```python
from build123d import *

# Parameters (mm, degrees)
CROQUIS1_R              = 3.25
SALIENTE_EXTRUIR1_DEPTH = 1.2
CROQUIS2_R              = 1.75
SALIENTE_EXTRUIR2_DEPTH = 22.1
REDONDEO2_R             = 0.4


with BuildPart() as part:
    # Croquis1 → Saliente-Extruir1 (new body)
    with BuildSketch(Plane.XY):
        Circle(CROQUIS1_R)
    extrude(amount=SALIENTE_EXTRUIR1_DEPTH)

    # Croquis2 → Saliente-Extruir2 (add)
    with BuildSketch(Plane(origin=(0, 0, 0), x_dir=(-1, 0, 0), z_dir=(0, 0, -1))):
        Circle(CROQUIS2_R)
    extrude(amount=SALIENTE_EXTRUIR2_DEPTH)

    # Redondeo2
    redondeo2_edges = [part.edges().sort_by_distance(p)[0] for p in [
        (-3.25, 0, 0),
        (-3.25, 0, 1.2),
    ]]
    fillet(redondeo2_edges, radius=REDONDEO2_R)


solid = part.part
```
The listing builds one solid part. Answer for the finished solid, in the listing's coordinates (mm). A direction names the side the tool comes from. Coordinates: 2 decimals unless noted, no trailing zeros. Write each loop counter-clockwise with the first axis right and the second up, starting at its lowest first coordinate (ties: lowest second). Pieces come first, ordered by that corner, then holes. Notation, with made-up numbers: (3.25, 48) - (60.25, 48) arc R27 cw to (60.25, 81) - close; hole circle Ø2 at (32, 55.25). An arc over 180 degrees is marked (long way). Return JSON: item names as keys, results as strings. Group by question number.
1. Which of the six approach directions +Z, -Z, +X, -X, +Y, -Y give full straight-line access (tool end or side, diameter ignored) to faces 1 (the cylindrical face through (-1.617, -0.67, -10.895)), 2 (the flat face through (0, 0, 1.2))?
2. Given pin 1 (2 mm diameter, centred on y = 0.5, z = -19.5, fed in from -X); pin 2 (3 mm diameter, centred on x = 2.5, z = -2.5, fed in from -Y); pin 3 (2 mm diameter, centred on y = 2, z = -1.5, fed in from -X), each flat-ended and moving along its own axis, determine where each tip first touches the part or whether it passes through.
3. A cutting plane is placed at A-A, the plane y = 0. Determine the outline of the cut face in (x, z).
4. A cutting plane is placed at C-C, the plane z = -10. Determine the outline of the cut face in (x, y).
5. Straight lines are drawn through the part: L1, parallel to Z at x = -2, y = -0.5; L2, parallel to X at y = -1.5, z = -6.75. For each, find the intervals that lie inside material, in ascending order.
Ans:
{
 "1": {"face 1": "-Z", "face 2": "+Z, +X, -X, +Y, -Y"},
 "2": {"pin 1": "x = -1.75", "pin 2": "y = -1.44", "pin 3": "x = -1.44"},
 "3": {"outline": "(-3.25, 0.4) arc R0.4 ccw to (-2.85, 0) - (-1.75, 0) - (-1.75, -22.1) - (1.75, -22.1) - (1.75, 0) - (2.85, 0) arc R0.4 ccw to (3.25, 0.4) - (3.25, 0.8) arc R0.4 ccw to (2.85, 1.2) - (-2.85, 1.2) arc R0.4 ccw to (-3.25, 0.8) - close"},
 "4": {"outline": "circle Ø3.5 at (0, 0)"},
 "5": {"L1": "0 to 1.2", "L2": "-0.9 to 0.9"}
}
